CAD build for the part. Positions are in the model's coordinates, mm. A direction names the side the tool comes from. Round coordinates to 2 decimals unless told otherwise and drop trailing zeros. Order: outer loops, then holes, each group sorted by start corner. A loop starts at its lowest first (then second) coordinate and runs counter-clockwise, first axis right, second up. Notation, with made-up numbers: M 36.5,20 L 44.5,20 A23 ccw 44.5,50 Z; hole C -12.5,-37 d3. An arc over 180 degrees is marked long. Answer as CSV lines item,"result". Start each with the question number.
```python
from build123d import *

# Parameters (mm, degrees)
SKIZZE1_W                       = 530
SKIZZE1_H                       = 320
AUFSATZ_LINEAR_AUSTRAGEN1_DEPTH = 53
FASE1_SIZE                      = 100
FASE1_SIZE2                     = 36.397023427
SKIZZE2_W                       = 90
SKIZZE2_H                       = 25
SCHNITT_LINEAR_AUSTRAGEN1_DEPTH = 530


with BuildPart() as part:
    # Skizze1 → Aufsatz-Linear austragen1 (new body)
    with BuildSketch(Plane(origin=(0, 0, 0), x_dir=(1, 0, 0), z_dir=(0, 1, 0))):
        Rectangle(SKIZZE1_W, SKIZZE1_H)
    extrude(amount=AUFSATZ_LINEAR_AUSTRAGEN1_DEPTH)

    # Fase1
    fase1_edges = [part.edges().sort_by_distance(p)[0] for p in [
        (0, 0, -160),
    ]]
    fase1_side = [part.faces().sort_by_distance(p)[0] for p in [
        (0, 0, 0),
    ]]
    chamfer(fase1_edges, length=FASE1_SIZE, length2=FASE1_SIZE2, reference=fase1_side[0])

    # Skizze2 → Schnitt-Linear austragen1 (cut)
    with BuildSketch(Plane(origin=(265, 0, 0), x_dir=(0, 0, -1), z_dir=(1, 0, 0))):
        with Locations((-115, 12.5)):
            Rectangle(SKIZZE2_W, SKIZZE2_H)
    extrude(amount=-SCHNITT_LINEAR_AUSTRAGEN1_DEPTH, mode=Mode.SUBTRACT)


solid = part.part
```
Q1. Band-saw the part on C-C, the plane z = -141. Write the cut outline in (x, y), then the cut area to 3 significant figures.
Q2. Band-saw the part on A-A, the plane x = 130.5. Write the cut outline in (y, z), then the cut area to 3 significant figures.
Q3. Band-saw the part on B-B, the plane y = 9.5. Write the cut outline in (x, z), then the cut area to 3 significant figures.
Q4. Drop flat-ended pins along their axis: P1, Ø7.5, axis at x = -97, y = 11.5, coming from the +Z side; P2, Ø8, axis at x = -172, z = 105, coming from the -Y side; P3, Ø8, axis at x = -114.5, z = -77, coming from the -Y side. Give the stop position or say it passes through.
Q5. Probe line 1 along Y through (x, z) = (-215, 76); line 2 along Y through (x, z) = (178.5, -140). List the from-to ranges inside material, lowest first. Write a range as from..to.
Q6. Tool access for faces 1 (the flat face through (4, 25, 116)), 2 (the flat face through (-4, 0, 4)): list every direction of +Z, -Z, +X, -X, +Y, -Y with a clear straight run to the whole face (end or side of a thin tool).
Answer:
1,outline,"M -265,29.48 L 265,29.48 L 265,53 L -265,53 Z"
1,area,"12,500 mm^2"
2,outline,"M 0,-60 L 36.4,-160 L 53,-160 L 53,160 L 25,160 L 25,70 L 0,70 Z"
2,area,"12,900 mm^2"
3,outline,"M -265,-86.1 L 265,-86.1 L 265,70 L -265,70 Z"
3,area,"82,700 mm^2"
4,P1,"stops at z = 70"
4,P2,"stops at y = 25"
4,P3,"stops at y = 4.73"
5,line 1,"y = 25..53"
5,line 2,"y = 29.12..53"
6,face 1,"+Z, +X, -X, -Y"
6,face 2,"+Z, -Z, +X, -X, -Y"
